from build123d import *

# Parameters (mm, degrees)
BOSS_EXTRUDE1_DEPTH = 5
SKETCH2_W           = 15
SKETCH2_H           = 0.5
CUT_EXTRUDE1_DEPTH  = 20.248376555
SKETCH3_R           = 1.5
SKETCH3_R_2         = 2
CUT_EXTRUDE2_DEPTH  = 18.036725037
SKETCH4_R           = 1.5
CUT_EXTRUDE3_DEPTH  = 19.145247312
FILLET1_R           = 0.25


with BuildPart() as part:
    # Sketch1 → Boss-Extrude1 (new, symmetric)
    with BuildSketch(Plane(origin=(0, 0, 0), x_dir=(1, 0, 0), z_dir=(0, 1, 0))):
        Polygon((-5, 2.5), (-4.196152423, 5.5), (4.196152423, 5.5), (5, 2.5), (15.5, 2.5), (15.5, -2.5), (-15.5, -2.5), (-15.5, 2.5), align=None)
    extrude(amount=BOSS_EXTRUDE1_DEPTH, both=True)

    # Sketch2 → Cut-Extrude1 (cut, through all)
    with BuildSketch(Plane(origin=(0, 5, 0), x_dir=(1, 0, 0), z_dir=(0, 1, 0))):
        with Locations((0, -2.25)):
            Rectangle(SKETCH2_W, SKETCH2_H)
    extrude(amount=-CUT_EXTRUDE1_DEPTH, mode=Mode.SUBTRACT)

    # Sketch3 → Cut-Extrude2 (cut, through all)
    with BuildSketch(Plane(origin=(0, 0, -2.5), x_dir=(-1, 0, 0), z_dir=(0, 0, -1))):
        Circle(SKETCH3_R)
        with Locations((12, 0)):
            Circle(SKETCH3_R_2)
        with Locations((-12, 0)):
            Circle(SKETCH3_R_2)
    extrude(amount=-CUT_EXTRUDE2_DEPTH, mode=Mode.SUBTRACT)

    # Sketch4 → Cut-Extrude3 (cut, through all)
    with BuildSketch(Plane(origin=(0, 0, -5.5), x_dir=(-1, 0, 0), z_dir=(0, 0, -1))):
        Circle(SKETCH4_R)
    extrude(amount=-CUT_EXTRUDE3_DEPTH, mode=Mode.SUBTRACT)

    # Fillet1
    fillet1_edges = [part.edges().sort_by_distance(p)[0] for p in [
        (15.5, -5, 0),
        (-11.5, -5, 2.5),
        (-15.5, -5, 0),
        (-10.25, -5, -2.5),
        (-11.5, 5, 2.5),
        (-5, 0, -2.5),
        (-4.196152423, 0, -5.5),
        (4.196152423, 0, -5.5),
        (5, 0, -2.5),
        (15.5, 0, -2.5),
        (15.5, 0, 2.5),
        (-15.5, 0, 2.5),
        (-15.5, 0, -2.5),
        (15.5, 5, 0),
        (10.25, 5, -2.5),
        (4.598076211, 5, -4),
        (11.5, -5, 2.5),
        (11.5, 5, 2.5),
        (0, 5, -5.5),
        (-7.5, -5, 2.25),
        (0, -5, 2),
        (7.5, -5, 2.25),
        (-7.5, 5, 2.25),
        (-4.598076211, 5, -4),
        (7.5, 5, 2.25),
        (0, 5, 2),
        (-10.25, 5, -2.5),
        (-4.598076211, -5, -4),
        (-15.5, 5, 0),
        (0, -5, -5.5),
        (4.598076211, -5, -4),
        (10.25, -5, -2.5),
    ]]
    fillet(fillet1_edges, radius=FILLET1_R)


solid = part.part
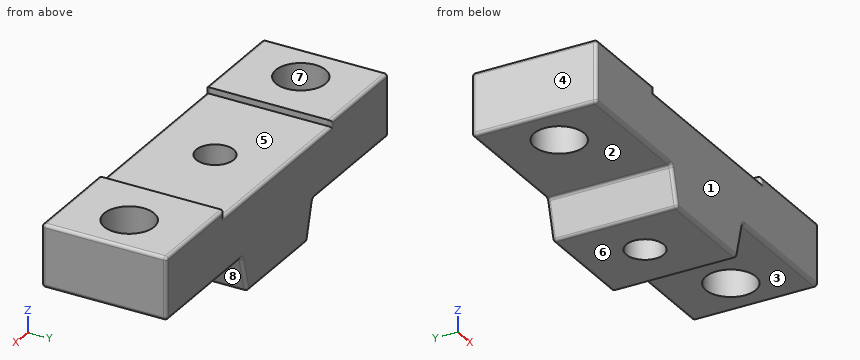
Part model, mm, in its own coordinate system. Face numbers are marked on the shaded views. A direction names the side the tool comes from. Round coordinates to 2 decimals unless told otherwise and drop trailing zeros. Write each loop counter-clockwise with the first axis right and the second up, starting at its lowest first coordinate (ties: lowest second). Pieces come first, ordered by that corner, then holes. Notation, with made-up numbers: M 36,54 L 55,54 A18 cw 55,84 Z; hole C 18.25,89.5 d7. An arc over 180 degrees is marked long. Return JSON: item names as keys, results as strings. Group by question number.
(1) Two-plate mould, pull along X, no slides. Class the marked faces 6, 7 and 8: +X half, -X half, draft (parallel to the pull), parting line (faces both ways), or undercut.
(2) Saw through at C-C on y = 3.5. Write the cut outline in (x, z), then the cut area to 3 significant figures.
(3) Saw through at B-B on x = 12. Write the cut outline in (y, z).
(4) Which spindle directions (+Z, -Z, +X, -X, +Y, -Y) get a long thin tool onto all of the face, cutting with end or side? Do the marked faces 1, 2, 3, 4 and 5. Say none if no direction does.
(5) Saw through at A-A on y = 0. Count the separate pieces of the cut face and the enclosed holes in it, then the cut area to 3 significant figures.
(6) Pin check, flat tips, straight feed: pin 1 Ø5 at (x, y) = (0, 0) entering from +Z; pin 2 Ø5 at (x, y) = (12, 0) entering from -Z; pin 3 Ø4.5 at (x, y) = (-12, 0) entering from +Z; pin 4 Ø2 at (x, z) = (-11.5, -4) entering from -Y. Stop position of each tip, or through.
(7) Drill centre lines: probe 1 along Y at (x, z) = (0, -1.5); probe 2 along Y at (x, z) = (12, 0); probe 3 along X at (y, z) = (1.75, -2.25). Where is each one in solid material? Low to high.
(8) Saw through at D-D on z = -0.25. Write the cut outline in (x, y), then the cut area to 3 significant figures.
Returned:
{
 "1": {"face 6": "draft", "face 7": "undercut", "face 8": "+X half"},
 "2": {"outline": "M -15.5,-2.25 A0.25 ccw -15.25,-2.5 L -5.19,-2.5 A0.25 cw -4.95,-2.69 L -4.25,-5.31 A0.25 ccw -4,-5.5 L 4,-5.5 A0.25 ccw 4.25,-5.31 L 4.95,-2.69 A0.25 cw 5.19,-2.5 L 15.25,-2.5 A0.25 ccw 15.5,-2.25 L 15.5,2.25 A0.25 ccw 15.25,2.5 L 7.5,2.5 L 7.5,2 L -7.5,2 L -7.5,2.5 L -15.25,2.5 A0.25 ccw -15.5,2.25 Z", "area": "175 mm²"},
 "3": {"outline": "M -5,-2.25 A0.25 ccw -4.75,-2.5 L -2,-2.5 L -2,2.5 L -4.75,2.5 A0.25 ccw -5,2.25 Z; M 2,-2.5 L 4.75,-2.5 A0.25 ccw 5,-2.25 L 5,2.25 A0.25 ccw 4.75,2.5 L 2,2.5 Z"},
 "4": {"face 1": "+Z, -Z, +X, -X, -Y", "face 2": "-Z, -X, +Y, -Y", "face 3": "-Z, +X, +Y, -Y", "face 4": "+Z, -Z, -X, +Y, -Y", "face 5": "+Z, +Y, -Y"},
 "5": {"separate pieces": "4", "enclosed holes": "0", "area": "113 mm²"},
 "6": {"pin 1": "z = 2", "pin 2": "z = -2.5", "pin 3": "z = 2.5", "pin 4": "through"},
 "7": {"probe 1": "-5 to -1.5, 1.5 to 5", "probe 2": "-5 to -2, 2 to 5", "probe 3": "-15.5 to -12.97, -11.03 to 11.03, 12.97 to 15.5"},
 "8": {"outline": "M -15.5,-4.75 A0.25 ccw -15.25,-5 L 15.25,-5 A0.25 ccw 15.5,-4.75 L 15.5,4.75 A0.25 ccw 15.25,5 L -15.25,5 A0.25 ccw -15.5,4.75 Z; hole C -12,0 d4; hole C 0,0 d3; hole C 12,0 d4", "area": "278 mm²"}
}
